Autodesk Inventor part; units mm, degrees
ref_plane "YZ Plane" through (0, 0, 0) normal (1, 0, 0) x (0, 1, 0)
ref_plane "XZ Plane" through (0, 0, 0) normal (0, 1, 0) x (-1, 0, 0)
ref_plane "XY Plane" through (0, 0, 0) normal (0, 0, 1) x (1, 0, 0)
sketch "스케치1" plane through (0, 0, 0) normal (0, 0, 1) x (1, 0, 0)
  line L0 (0, 0) -> (150, 0)
  line L1 (150, 0) -> (150, 60)
  line L2 (150, 60) -> (0, 60)
  line L3 (0, 60) -> (0, 0)
  circle A0 centre (20, 30) radius 2.5
  circle A1 centre (20, 10) radius 2.5
  circle A2 centre (130, 30) radius 2.5
  circle A3 centre (130, 10) radius 2.5
  line L4 (10, 60) -> (10, 0)
  line L5 (20, 60) -> (20, 50)
  line L6 (20, 50) -> (10, 50)
  line L7 (20, 50) -> (20, 25)
  line L8 (20, 25) -> (10, 25)
  line L9 (10, 15) -> (0, 15)
  line L10 (20, 40) -> (150, 40)
  point P0 (20, 27.5)
  point P1 (20, 32.5)
  dimension "d0" = 5
  dimension "d1" = 30
  dimension "d2" = 20
  dimension "d3" = 20
  dimension "d4" = 150
  dimension "d5" = 20
  dimension "d6" = 60
  dimension "d7" = 10
  dimension "d8" = 10
  dimension "d9" = 10
  dimension "d10" = 10
  dimension "d11" = 25
  dimension "d16" = 10
  dimension "d19" = 20
extrude "돌출1" add sketch "스케치1" against normal blind 10 contours L3 L9 L4 L0 | L4 L8 L7 A0 L10 L1 L0 | L3 L2 L4 L9 | L10 L7 L5 L2 L1 | L4 L6 L7 A0 L8
extrude "돌출2" add sketch "스케치1" along normal blind 75 contours L3 L2 L4 L9 | L4 L6 L7 A0 L8
sketch "스케치2" plane through (0, 0, -10) normal (-1, 0, 0) x (0, 0, 1)
  line L0 (0, 60) -> (85, 60)
  line L1 (0, 0) -> (0, 60)
  line L2 (10, 0) -> (0, 0)
  line L3 (10, 15) -> (10, 0)
  line L4 (10, 15) -> (85, 15)
  line L5 (85, 60) -> (85, 15)
  line L6 (85, 15) -> (10, 0)
extrude "돌출3" add sketch "스케치2" against normal up to surface (10 mm away) contours L6 L3 L4
extrude "돌출4" add sketch "스케치1" along normal blind 15 contours L10 L7 L5 L2 L1
properties part number "NewModuleConnectorLeft_3D 인쇄"
Model file for the job. Use its own axes, mm. A direction names the side the tool comes from. Round coordinates to 2 decimals unless told otherwise and drop trailing zeros. Order: outer loops, then holes, each group sorted by start corner. A loop starts at its lowest first (then second) coordinate and runs counter-clockwise, first axis right, second up.
(1) Pin check, flat tips, straight feed: pin 1 (11 mm diameter, centred on x = 12.5, z = 48.5, fed in from -Y); pin 2 (5 mm diameter, centred on y = 38, z = 51.5, fed in from +X); pin 3 (5 mm diameter, centred on y = 55, z = 32.5, fed in from +X). Stop position of each tip, or through.
(2) Pull direction X, two halves, no side cores. Call faces 6 (the face through (15, 50, 33)), 7 (the face through (10, 15, 29)), 8 (the face through (84, 40, 7)): released by +X, released by -X, zero draft, split by the parting line, or undercut.
(3) 3-axis set-ups, long thin cutter, end or side, ignore diameter. For faces 1 (the face through (84, 50, 15)), 2 (the face through (10, 55, 33)), 3 (the face through (15, 25, 37)), 4 (the face through (74, 30, -10)), 5 (the face through (132.31, 9.04, -4.93)): which of +Z, -Z, +X, -X, +Y, -Y reach the whole face in a straight line?
(4) Band-saw the part on C-C (y = 30). List the corners of the cut face in (x, z).
(5) Band-saw the part on A-A (x = 130). List the corners of the cut face in (y, z), then the cut area to 3 significant figures.
(6) Drill centre lines: line 1 (Y direction, x = 130, z = -3); line 2 (X direction, y = 43, z = 45.5); line 3 (Z direction, x = 100, y = 37.5). Where is each one in solid material? Low to high.
(7) Band-saw the part on B-B (y = 54). List the corners of the cut face in (x, z), then the cut area to 3 significant figures.
(8) Band-saw the part on D-D (z = 54). List the corners of the cut face in (x, y), then the cut area to 3 significant figures.
Verdict:
1. pin 1: stops at y = 8.72
1. pin 2: stops at x = 20
1. pin 3: stops at x = 10
2. face 6: undercut
2. face 7: released by +X
2. face 8: zero draft
3. face 1: +Z, +X, +Y, -Y
3. face 2: +Z, -Z, +Y
3. face 3: +Z, +X, -Y
3. face 4: -Z, +X, -X, +Y, -Y
3. face 5: +Z, -Z
4. outline: (0, -10) - (17.5, -10) - (17.5, 75) - (0, 75) - close; (22.5, -10) - (127.5, -10) - (127.5, 0) - (22.5, 0) - close; (132.5, -10) - (150, -10) - (150, 0) - (132.5, 0) - close
5. outline: (0, -10) - (7.5, -10) - (7.5, 0) - (0, 0) - close; (12.5, -10) - (27.5, -10) - (27.5, 0) - (12.5, 0) - close; (32.5, -10) - (60, -10) - (60, 15) - (40, 15) - (40, 0) - (32.5, 0) - close
5. area: 800 mm2
6. line 1: y = 0 to 7.5, 12.5 to 27.5, 32.5 to 60
6. line 2: x = 0 to 20
6. line 3: z = -10 to 0
7. outline: (0, -10) - (10, -10) - (10, 75) - (0, 75) - close; (20, -10) - (150, -10) - (150, 15) - (20, 15) - close
7. area: 4,100 mm2
8. outline: (0, 10.8) - (10, 10.8) - (10, 25) - (20, 25) - (20, 27.5) arc R2.5 cw to (20, 32.5) - (20, 50) - (10, 50) - (10, 60) - (0, 60) - close
8. area: 732 mm2
